Part model, mm, in its own coordinate system. Face numbers are marked on the shaded views. A direction names the side the tool comes from. Round coordinates to 2 decimals unless told otherwise and drop trailing zeros. Write each loop counter-clockwise with the first axis right and the second up, starting at its lowest first coordinate (ties: lowest second). Pieces come first, ordered by that corner, then holes.
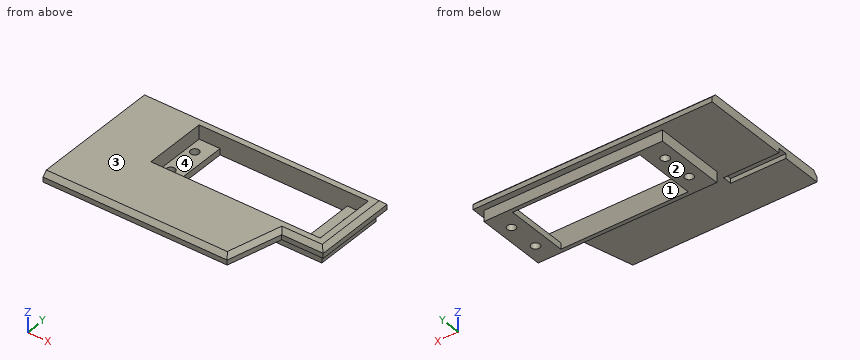
from build123d import *

# Parameters (mm, degrees)
BOSS_EXTRUDE1_DEPTH = 3
CUT_EXTRUDE1_REACH  = 82.709
CUT_EXTRUDE2_REACH  = 82.709
CUT_EXTRUDE3_DEPTH  = 49.851933985
CUT_EXTRUDE4_REACH  = 63.973
SKETCH9_W           = 57.5
SKETCH9_H           = 22.75
BOSS_EXTRUDE2_DEPTH = 3.5
SKETCH13_W          = 54.5
SKETCH13_H          = 20.25
CUT_EXTRUDE6_DEPTH  = 4.5
SKETCH14_W          = 41
SKETCH14_H          = 20.25
CUT_EXTRUDE7_DEPTH  = 2
CUT_EXTRUDE8_REACH  = 49.521
SKETCH15_R          = 1.375
SKETCH16_W          = 17.807241949
SKETCH16_H          = 3
CUT_EXTRUDE9_DEPTH  = 1.5


with BuildPart() as part:
    # Sketch4 → Boss-Extrude1 (new body)
    with BuildSketch(Plane.XY):
        Polygon((22.874373936, -2.75), (36.232991843, -2.75), (36.232991843, 24), (-40.767008157, 24), (-40.767008157, -20), (18.555957827, -20), align=None)
    extrude(amount=BOSS_EXTRUDE1_DEPTH)

    # Sketch5 → Cut-Extrude1 (cut, up to next)
    with BuildSketch(Plane(origin=(36.232991843, 0, 0), x_dir=(0, 0, -1), z_dir=(1, 0, 0)), mode=Mode.PRIVATE) as cut_extrude1_sk1:
        Polygon((-3, 22.585786438), (-1.585786438, 24), (-3, 24), align=None)
    cut_extrude1_tool1 = extrude(cut_extrude1_sk1.sketch, amount=-CUT_EXTRUDE1_REACH, mode=Mode.PRIVATE) & part.part
    # Sketch5 → Cut-Extrude1 (cut, up to next)
    with BuildSketch(Plane(origin=(36.232991843, 0, 0), x_dir=(0, 0, -1), z_dir=(1, 0, 0)), mode=Mode.PRIVATE) as cut_extrude1_sk2:
        Polygon((-3, -18.585786438), (-1.585786438, -20), (-3, -20), align=None)
    cut_extrude1_tool2 = extrude(cut_extrude1_sk2.sketch, amount=-CUT_EXTRUDE1_REACH, mode=Mode.PRIVATE) & part.part
    add(cut_extrude1_tool1.solids().sort_by_distance((36.232992, 23.528595, 2.528595))[0], mode=Mode.SUBTRACT)
    add(cut_extrude1_tool2.solids().sort_by_distance((36.232992, -19.528595, 2.528595))[0], mode=Mode.SUBTRACT)

    # Cut-Extrude2: up to this plane
    cut_extrude2_end = Plane(origin=(18.555957827, -20, 3), z_dir=(-0.9700641682071632, 0.24284873802543147, 0))
    # Sketch5<4> → Cut-Extrude2 (cut, up to the surface)
    with BuildSketch(Plane(origin=(36.232991843, 0, 0), x_dir=(0, 0, -1), z_dir=(1, 0, 0)), mode=Mode.PRIVATE) as cut_extrude2_sk1:
        Polygon((-1.585786438, -2.75), (-3, -1.335786438), (-3, -2.75), align=None)
    cut_extrude2_tool1 = split(extrude(cut_extrude2_sk1.sketch, amount=-CUT_EXTRUDE2_REACH, mode=Mode.PRIVATE), bisect_by=cut_extrude2_end, keep=Keep.BOTH, mode=Mode.PRIVATE)
    add(cut_extrude2_tool1.solids().sort_by_distance((36.232992, -2.278595, 2.528595))[0], mode=Mode.SUBTRACT)

    # Sketch7 → Cut-Extrude3 (cut, through all)
    with BuildSketch(Plane.XZ.offset(2.75)):
        Polygon((36.232991843, 1.585786438), (34.818778281, 3), (36.232991843, 3), align=None)
    extrude(amount=-CUT_EXTRUDE3_DEPTH, mode=Mode.SUBTRACT)

    # Cut-Extrude4: up to this plane
    cut_extrude4_end = Plane(origin=(21.020533502, -2.167893219, 2.167893219), z_dir=(0, 0.7071067811865472, -0.707106781186548))
    # Sketch8 → Cut-Extrude4 (cut, up to the surface)
    with BuildSketch(Plane.XZ.offset(20), mode=Mode.PRIVATE) as cut_extrude4_sk1:
        Polygon((17.141744264, 3), (18.555957827, 3), (18.555957827, 1.585786438), align=None)
    cut_extrude4_tool1 = split(extrude(cut_extrude4_sk1.sketch, amount=CUT_EXTRUDE4_REACH, dir=(0.242848738025, 0.970064168207, 0), mode=Mode.PRIVATE), bisect_by=cut_extrude4_end, keep=Keep.BOTH, mode=Mode.PRIVATE)
    add(cut_extrude4_tool1.solids().sort_by_distance((18.084553, -20, 2.528595))[0], mode=Mode.SUBTRACT)

    # Sketch9 → Boss-Extrude2 (add)
    with BuildSketch(Plane.XY):
        with Locations((5.482991843, 10.625)):
            Rectangle(SKETCH9_W, SKETCH9_H)
    extrude(amount=-BOSS_EXTRUDE2_DEPTH)

    # Sketch13 → Cut-Extrude6 (cut)
    with BuildSketch(Plane.XY.offset(3)):
        with Locations((5.482991843, 10.625)):
            Rectangle(SKETCH13_W, SKETCH13_H)
    extrude(amount=-CUT_EXTRUDE6_DEPTH, mode=Mode.SUBTRACT)

    # Sketch14 → Cut-Extrude7 (cut)
    with BuildSketch(Plane.XY.offset(-1.5)):
        with Locations((5.482991843, 10.625)):
            Rectangle(SKETCH14_W, SKETCH14_H)
    extrude(amount=-CUT_EXTRUDE7_DEPTH, mode=Mode.SUBTRACT)

    # Sketch15 → Cut-Extrude8 (cut, up to next)
    with BuildSketch(Plane.XY.offset(-1.5), mode=Mode.PRIVATE) as cut_extrude8_sk1:
        with Locations((30.232991843, 15.675)):
            Circle(SKETCH15_R)
    cut_extrude8_tool1 = extrude(cut_extrude8_sk1.sketch, amount=-CUT_EXTRUDE8_REACH, mode=Mode.PRIVATE) & part.part
    # Sketch15 → Cut-Extrude8 (cut, up to next)
    with BuildSketch(Plane.XY.offset(-1.5), mode=Mode.PRIVATE) as cut_extrude8_sk2:
        with Locations(Location((30.232991843, 5.575, 0), (0, 0, 180))):
            Circle(SKETCH15_R)
    cut_extrude8_tool2 = extrude(cut_extrude8_sk2.sketch, amount=-CUT_EXTRUDE8_REACH, mode=Mode.PRIVATE) & part.part
    # Sketch15 → Cut-Extrude8 (cut, up to next)
    with BuildSketch(Plane.XY.offset(-1.5), mode=Mode.PRIVATE) as cut_extrude8_sk3:
        with Locations((-19.267008157, 5.575)):
            Circle(SKETCH15_R)
    cut_extrude8_tool3 = extrude(cut_extrude8_sk3.sketch, amount=-CUT_EXTRUDE8_REACH, mode=Mode.PRIVATE) & part.part
    # Sketch15 → Cut-Extrude8 (cut, up to next)
    with BuildSketch(Plane.XY.offset(-1.5), mode=Mode.PRIVATE) as cut_extrude8_sk4:
        with Locations(Location((-19.267008157, 15.675, 0), (0, 0, 180))):
            Circle(SKETCH15_R)
    cut_extrude8_tool4 = extrude(cut_extrude8_sk4.sketch, amount=-CUT_EXTRUDE8_REACH, mode=Mode.PRIVATE) & part.part
    add(cut_extrude8_tool1.solids().sort_by_distance((30.232992, 15.675, -1.5))[0], mode=Mode.SUBTRACT)
    add(cut_extrude8_tool2.solids().sort_by_distance((30.232992, 5.575, -1.5))[0], mode=Mode.SUBTRACT)
    add(cut_extrude8_tool3.solids().sort_by_distance((-19.267008, 5.575, -1.5))[0], mode=Mode.SUBTRACT)
    add(cut_extrude8_tool4.solids().sort_by_distance((-19.267008, 15.675, -1.5))[0], mode=Mode.SUBTRACT)

    # Sketch16 → Cut-Extrude9 (cut)
    with BuildSketch(Plane(origin=(0, 0, 0), x_dir=(-1, 0, 0), z_dir=(0, 0, -1))):
        with Locations((31.863387182, -5.5)):
            Rectangle(SKETCH16_W, SKETCH16_H)
    extrude(amount=-CUT_EXTRUDE9_DEPTH, mode=Mode.SUBTRACT)


solid = part.part
Q1. Wall check: line 1 (X direction, y = 12.5, z = -0.5); line 2 (X direction, y = 6, z = 0.75); line 3 (Y direction, x = -8.5, z = 1.5). Give the ranges that are in metal, low to high.
Q2. Drop flat-ended pins along their axis: P1, Ø3, axis at x = 25, z = -2.5, coming from the -Y side; P2, Ø2, axis at y = 8.5, z = -2, coming from the -X side; P3, Ø3.5, axis at x = 28.5, y = 11.5, coming from the +Z side; P4, Ø3, axis at y = -5.5, z = -2.5, coming from the +X side. Give the stop position or say it passes through.
Q3. Saw through at C-C, the plane z = 0.75. Write the cut outline in (x, y).
Q4. Two-plate mould, pull along Y, no slides. Class the marked faces 1 and 2: released by +Y, released by -Y, zero draft, split by the parting line, or undercut.
Q5. Saw through at A-A, the plane x = 10. Write the cut outline in (y, z), and give its area (3 significant figures).
Q6. Tool access for the marked faces 3 and 4: list every direction of +Z, -Z, +X, -X, +Y, -Y with a clear straight run to the whole face (end or side of a thin tool).
Q7. Saw through at D-D, the plane z = -2.75. Write the cut outline in (x, y) (3 decimals).
Q8. Saw through at B-B, the plane y = 3. Write the cut outline in (x, z).
Computed:
1. line 1: x = -23.27 to -21.77, 32.73 to 34.23
1. line 2: x = -40.77 to -21.77, 32.73 to 36.23
1. line 3: y = -20 to 0.5, 20.75 to 24
2. P1: stops at y = -0.75
2. P2: stops at x = -23.27
2. P3: stops at z = -1.5
2. P4: passes through
3. outline: (-40.77, -20) - (18.56, -20) - (22.87, -2.75) - (36.23, -2.75) - (36.23, 24) - (-40.77, 24) - (-40.77, -4) - (-22.96, -4) - (-22.96, -7) - (-40.77, -7) - close; hole (-21.77, 0.5) - (32.73, 0.5) - (32.73, 20.75) - (-21.77, 20.75) - close
4. face 1: undercut
4. face 2: zero draft
5. outline: (-20, 0) - (-0.75, 0) - (-0.75, -3.5) - (0.5, -3.5) - (0.5, 3) - (-18.59, 3) - (-20, 1.59) - close; (20.75, -3.5) - (22, -3.5) - (22, 0) - (24, 0) - (24, 1.59) - (22.59, 3) - (20.75, 3) - close
5. area: 78.0 mm2
6. face 3: +Z, +X, -X, +Y, -Y
6. face 4: +Z
7. outline: (-23.267, -0.75) - (34.233, -0.75) - (34.233, 22) - (-23.267, 22) - close; hole circle Ø2.75 at (-19.267, 5.575); hole circle Ø2.75 at (-19.267, 15.675); hole (-15.017, 0.5) - (25.983, 0.5) - (25.983, 20.75) - (-15.017, 20.75) - close; hole circle Ø2.75 at (30.233, 5.575); hole circle Ø2.75 at (30.233, 15.675)
8. outline: (-40.77, 0) - (-23.27, 0) - (-23.27, -3.5) - (-15.02, -3.5) - (-15.02, -1.5) - (-21.77, -1.5) - (-21.77, 3) - (-40.77, 3) - close; (25.98, -3.5) - (34.23, -3.5) - (34.23, 0) - (36.23, 0) - (36.23, 1.59) - (34.82, 3) - (32.73, 3) - (32.73, -1.5) - (25.98, -1.5) - close
